Could you check a few things on this model? Use its own coordinates, in mm. A direction names the side the tool comes from. Coordinates: 2 decimals unless noted, no trailing zeros. Return JSON: item names as keys, results as strings. Group by question number.
from build123d import *

# Parameters (mm, degrees)
F1_DEPTH = 1


with BuildPart() as f1:
    # F0 (on Top) → F1 (new body)
    with BuildSketch(Plane.XY):
        with BuildLine():
            Line((-12.5, 5), (-20, 5))
            Line((-20, 5), (-25, 5))
            Line((-25, 5), (-25, -5))
            Line((-25, -5), (-20, -5))
            Line((-20, -5), (-12.5, -5))
            add(Edge.make_bspline(
                [(-5, -1), (-7.8716344223, -1.8257793632), (-10.1858172112, -3.4128896816), (-12.5, -5)],
                knots=[0.6758143524, 0.6758143524, 0.6758143524, 0.6758143524, 1, 1, 1, 1], degree=3))
            add(Edge.make_bspline(
                [(5, -1), (1.8852751504, -0.1043165234), (-1.8852751504, -0.1043165234), (-5, -1)],
                knots=[0.3241856476, 0.3241856476, 0.3241856476, 0.3241856476, 0.6758143524, 0.6758143524, 0.6758143524, 0.6758143524], degree=3))
            add(Edge.make_bspline(
                [(12.5, -5), (10.1858172112, -3.4128896816), (7.8716344223, -1.8257793632), (5, -1)],
                knots=[0, 0, 0, 0, 0.3241856476, 0.3241856476, 0.3241856476, 0.3241856476], degree=3))
            Line((12.5, -5), (20, -5))
            Line((20, -5), (25, -5))
            Line((25, -5), (25, 5))
            Line((25, 5), (20, 5))
            Line((20, 5), (12.5, 5))
            add(Edge.make_bspline(
                [(5, 1), (7.8716344223, 1.8257793632), (10.1858172112, 3.4128896816), (12.5, 5)],
                knots=[0.6758143524, 0.6758143524, 0.6758143524, 0.6758143524, 1, 1, 1, 1], degree=3))
            add(Edge.make_bspline(
                [(-5, 1), (-1.8852751504, 0.1043165234), (1.8852751504, 0.1043165234), (5, 1)],
                knots=[0.3241856476, 0.3241856476, 0.3241856476, 0.3241856476, 0.6758143524, 0.6758143524, 0.6758143524, 0.6758143524], degree=3))
            add(Edge.make_bspline(
                [(-12.5, 5), (-10.1858172112, 3.4128896816), (-7.8716344223, 1.8257793632), (-5, 1)],
                knots=[0, 0, 0, 0, 0.3241856476, 0.3241856476, 0.3241856476, 0.3241856476], degree=3))
        make_face()
        with BuildLine():
            Line((5, 1), (-5, 1))
            add(Edge.make_bspline(
                [(-5, 1), (-1.8852751504, 0.1043165234), (1.8852751504, 0.1043165234), (5, 1)],
                knots=[0.3241856476, 0.3241856476, 0.3241856476, 0.3241856476, 0.6758143524, 0.6758143524, 0.6758143524, 0.6758143524], degree=3))
        make_face()
        with BuildLine():
            add(Edge.make_bspline(
                [(5, -1), (1.8852751504, -0.1043165234), (-1.8852751504, -0.1043165234), (-5, -1)],
                knots=[0.3241856476, 0.3241856476, 0.3241856476, 0.3241856476, 0.6758143524, 0.6758143524, 0.6758143524, 0.6758143524], degree=3))
            Line((-5, -1), (5, -1))
        make_face()
    extrude(amount=F1_DEPTH)


solid = f1.part
Q1. I need wall thicknesses on line 1 along X through (y, z) = (3.75, 0.7); line 2 along Y through (x, z) = (4.5, 0.1); line 3 along X through (y, z) = (-2.5, 0.4). Which ranges of each line are inside material? Lowest first, please. Write a range as from..to.
Q2. On a 3-axis mill with a long thin cutter (end or side, diameter ignored), from which of +Z, -Z, +X, -X, +Y, -Y can I reach the whole of each face in a straight line? I mean faces 5 (the flat face through (-0.1, -1, 0.5)), 6 (the flat face through (0, 0, 1)). Say none if no direction works.
Q3. I'm going to push flat-ended pins straight in: pin 1 Ø0.5 at (x, z) = (-0.5, 0.5) entering from -Y; pin 2 Ø1 at (x, y) = (-2.5, -2.5) entering from +Z (3 decimals). Where does each tip first touch, or does it pass through?
Q4. We'd pull the mould along X, two halves only. Please class faces 1 (the flat face through (25, -0.1, 0.5)), 2 (the flat face through (-25, 0.1, 0.5)), 3 (the flat face through (0, 0, 0)), 4 (the flat face through (0.1, 1, 0.5)): pulls with the +X half, pulls with the -X half, needs draft (parallel to the pull), parting line crosses it, or undercut.
Response values:
{
 "1": {"line 1": "x = -25..-10.65, 10.65..25", "line 2": "y = -1..1", "line 3": "x = -25..-8.57, 8.57..25"},
 "2": {"face 5": "+Z, -Z, -Y", "face 6": "+Z, +X, -X, +Y, -Y"},
 "3": {"pin 1": "stops at y = -1", "pin 2": "passes through"},
 "4": {"face 1": "pulls with the +X half", "face 2": "pulls with the -X half", "face 3": "needs draft", "face 4": "undercut"}
}
